```python
from build123d import *

# Parameters (mm, degrees)
BASPROSKE_W        = 11.5
BASPROSKE_H        = 6.6
TOOTHCUT_DEPTH     = 15.811144453
TEETHCUTS_COUNT    = 10
TEETHCUTS_ANGLE    = 324
BORSKE_R           = 1.5
BORE_DEPTH         = 50.0003556
SKETCH2_R          = 3.3
CUT_EXTRUDE1_DEPTH = 5.5
CUT_EXTRUDE2_START = -3.3
SKETCH3_R          = 3.3
CUT_EXTRUDE2_DEPTH = 3.3
SKETCH4_R          = 1.65
CUT_EXTRUDE3_DEPTH = 13.294146319
CHAMFER1_SIZE      = 0.3


with BuildPart() as part:
    # BasProSke → Base-Revolve (revolve)
    with BuildSketch(Plane(origin=(0, 0, 0), x_dir=(1, 0, 0), z_dir=(0, 1, 0)), mode=Mode.PRIVATE) as base_revolve_sk:
        with Locations((5.75, 3.3)):
            Rectangle(BASPROSKE_W, BASPROSKE_H)
    revolve(base_revolve_sk.sketch.rotate(Axis((-10, 0, 0), (1, 0, 0)), 180), axis=Axis((-10, 0, 0), (1, 0, 0)))

    # TooCutSke → ToothCut (cut, through all)
    with BuildSketch(Plane(origin=(0, 0, 0), x_dir=(0, 0, -1), z_dir=(1, 0, 0))):
        with BuildLine():
            ThreePointArc((0.749284073, 4.055360573), (0, 4.124), (-0.749284073, 4.055360573))
            ThreePointArc((-0.749284073, 4.055360573), (-0.916574147, 5.384052291), (-1.823298638, 6.369576692))
            ThreePointArc((-1.823298638, 6.369576692), (0, 6.6254), (1.823298638, 6.369576692))
            ThreePointArc((1.823298638, 6.369576692), (0.916574147, 5.384052291), (0.749284073, 4.055360573))
        make_face()
    toothcut = extrude(amount=TOOTHCUT_DEPTH, mode=Mode.SUBTRACT)

    # TeethCuts: ToothCut ×10 about axis
    teethcuts_axis = Axis((-10, 0, 0), (1, 0, 0))
    for i in range(1, TEETHCUTS_COUNT):
        add(toothcut.rotate(teethcuts_axis, i * TEETHCUTS_ANGLE / (TEETHCUTS_COUNT - 1)), mode=Mode.SUBTRACT)

    # BorSke → Bore (cut, symmetric)
    with BuildSketch(Plane(origin=(0, 0, 0), x_dir=(0, 0, -1), z_dir=(1, 0, 0))):
        with Locations(Location((0, 0, 0), (0, 0, 180))):
            Circle(BORSKE_R)
    extrude(amount=BORE_DEPTH, both=True, mode=Mode.SUBTRACT)

    # Sketch2 → Cut-Extrude1 (cut)
    with BuildSketch(Plane(origin=(11.5, 0, 0), x_dir=(0, 0, -1), z_dir=(1, 0, 0))):
        Circle(SKETCH2_R)
    extrude(amount=-CUT_EXTRUDE1_DEPTH, mode=Mode.SUBTRACT)

    # Sketch3 → Cut-Extrude2 (cut)
    with BuildSketch(Plane.ZY.offset(CUT_EXTRUDE2_START)):
        with Locations(Location((0, 0, 0), (0, 0, 180))):
            Circle(SKETCH3_R)
    extrude(amount=CUT_EXTRUDE2_DEPTH, mode=Mode.SUBTRACT)

    # Sketch4 → Cut-Extrude3 (cut, through all)
    with BuildSketch(Plane.ZY.offset(-3.3)):
        Circle(SKETCH4_R)
    extrude(amount=-CUT_EXTRUDE3_DEPTH, mode=Mode.SUBTRACT)

    # Chamfer1
    chamfer1_edges = [part.edges().sort_by_distance(p)[0] for p in [
        (11.5, 0, 3.3),
        (0, 0, 3.3),
    ]]
    chamfer(chamfer1_edges, length=CHAMFER1_SIZE)


solid = part.part
```
Geometry: final body of the model. Coordinates: model frame, mm. A direction names the side the tool comes from. Round coordinates to 2 decimals unless told otherwise and drop trailing zeros. Loops run counter-clockwise (first coordinate to the right, second up) from the corner with the lowest first, then second, coordinate; pieces in that order, holes last. Notation, with made-up numbers: (27.5, 49.25) -> (81.5, 49.25) arc R18 ccw to (81.5, 67.25) -> close; hole circle Ø4 at (-14.75, -38.75). An arc over 180 degrees is marked (long way). Use one line per item in the form item = value. Start each with the question number.
1) Section A-A on z = 0. Output: boundary loops of the cut face in (x, y), then the cut area to 3 significant figures.
2) Line query: L1, parallel to Y at x = 4.5, z = 0; L2, parallel to Z at x = 5, y = 3.5; L3, parallel to Z at x = 4.25, y = -3. Output: solid intervals per line, ascending.
3) Access query for faces 1 (the cylindrical face through (1.82, -2.23, 2.43)), 2 (the flat face through (6, -1, 2)). Directions: +Z, -Z, +X, -X, +Y, -Y. A direction counts if a zero-diameter tool reaches every point of the face in a straight line with its end or side. Return the directions, or none.
4) First-contact query: P1, Ø1, axis at x = 2.5, y = 3.5, coming from the +Z side; P2, Ø6, axis at x = 5.5, z = 4.5, coming from the +Y side; P3, Ø4, axis at x = 9.5, y = -2.5, coming from the -Z side. Flat tips, straight axial feed; report the tip coordinate or a pass-through.
5) Section B-B on y = 0. Output: boundary loops of the cut face in (x, z).
Response:
q1.outline = (0, -4.12) -> (11.5, -4.12) -> (11.5, -3.6) -> (11.2, -3.3) -> (6, -3.3) -> (6, -1.65) -> (3.3, -1.65) -> (3.3, -3.3) -> (0.3, -3.3) -> (0, -3.6) -> close; (0, 3.6) -> (0.3, 3.3) -> (3.3, 3.3) -> (3.3, 1.65) -> (6, 1.65) -> (6, 3.3) -> (11.2, 3.3) -> (11.5, 3.6) -> (11.5, 4.12) -> (0, 4.12) -> close
q1.area = 27.7 mm^2
q2.L1 = -4.12 to -1.65, 1.65 to 4.12
q2.L2 = -5.44 to -3.47, -2.18 to 2.18, 3.47 to 5.44
q2.L3 = -5.22 to -3.07, -2.83 to 2.83, 3.07 to 5.22
q3.face_1 = -X
q3.face_2 = +X
q4.P1 = 5.49
q4.P2 = 6.35
q4.P3 = -6.26
q5.outline = (0, -6.6) -> (11.5, -6.6) -> (11.5, -3.6) -> (11.2, -3.3) -> (6, -3.3) -> (6, -1.65) -> (3.3, -1.65) -> (3.3, -3.3) -> (0.3, -3.3) -> (0, -3.6) -> close; (0, 3.6) -> (0.3, 3.3) -> (3.3, 3.3) -> (3.3, 1.65) -> (6, 1.65) -> (6, 3.3) -> (11.2, 3.3) -> (11.5, 3.6) -> (11.5, 6.6) -> (0, 6.6) -> close
